```python
from build123d import *

# Parameters (mm, degrees)
F3_R = 5


with BuildPart() as f2:
    # F0 (on Front) → F2 (revolve)
    with BuildSketch(Plane.XZ):
        Polygon((-29.959241, 0), (0, 0), (0, 60.040765), (-16.230465, 27.513588), (-10.394023, 27.513588), (-10.394023, 22.020024), (-18.971652, 22.020024), align=None)
    revolve(axis=Axis((0, 0, 23.967392), (0, 0, -1)))

    # F3
    f3_edges = [f2.edges().sort_by_distance(p)[0] for p in [
        (29.959241, 0, 0),
    ]]
    fillet(f3_edges, radius=F3_R)


solid = f2.part
```
Here's how the part is built. I have some questions about the finished solid (model axes, mm). A direction names the side the tool comes from. Round coordinates to 2 decimals unless told otherwise and drop trailing zeros. Order: outer loops, then holes, each group sorted by start corner. A loop starts at its lowest first (then second) coordinate and runs counter-clockwise, first axis right, second up. Notation, with made-up numbers: (61.25, 72) -> (115.25, 72) arc R29 cw to (115.25, 97) -> close; hole circle Ø7 at (42.25, 29.5). An arc over 180 degrees is marked (long way). Use a Markdown table: item, result. Add a question column.
(1) For pin 1 Ø4 at (x, y) = (1.5, 9) entering from +Z; pin 2 Ø6 at (y, z) = (-19.5, 32) entering from -X; pin 3 Ø2 at (y, z) = (-9, 17.5) entering from +X; pin 4 Ø6 at (x, y) = (-12, 7) entering from +Z, each with a flat end and sliding along its axis, tell me the tip position at first contact or that it passes through.
(2) Suppose I cut it at A-A, the plane z = 38.5. Please give me the cut outline in (x, y), and give its area (3 significant figures).
(3) If we mould it in two halves opening along Z, with no side actions, what happens to faces 1 (the face through (0, -11, 27.514)), 2 (the face through (1.393, -6.273, 47.164)), 3 (the face through (0, 0, 0))? For each: released by +Z, released by -Z, zero draft, split by the parting line, or undercut.
(4) For faces 4 (the face through (4.213, -18.971, 21.095)), 5 (the face through (-9.6, -3.98, 24.73)), which set-ups out of +Z, -Z, +X, -X, +Y, -Y let a thin tool reach every point of the face, with its end or its side?
(5) I need wall thicknesses on line 1 along Z through (x, y) = (2.5, 15.5); line 2 along Z through (x, y) = (17.5, -3); line 3 along X through (y, z) = (9, 32.5). Which ranges of each line are inside material? Lowest first, please.
Verdict:
| question | item | result |
|---|---|---|
| 1 | pin 1 | z = 45.76 |
| 1 | pin 2 | through |
| 1 | pin 3 | x = 19.93 |
| 1 | pin 4 | z = 38.21 |
| 2 | outline | circle Ø21.5 at (0, 0) |
| 2 | area | 363 mm2 |
| 3 | face 1 | undercut |
| 3 | face 2 | released by +Z |
| 3 | face 3 | released by -Z |
| 4 | face 4 | +Z |
| 4 | face 5 | none |
| 5 | line 1 | 0 to 22.02, 27.51 to 28.58 |
| 5 | line 2 | 0 to 22.02 |
| 5 | line 3 | -10.39 to 10.39 |
